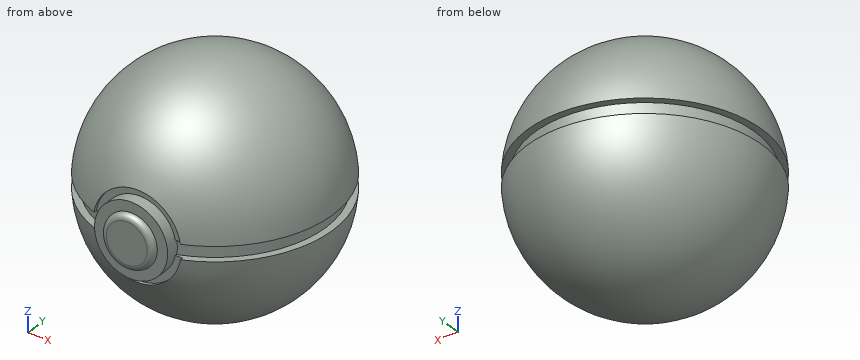
from build123d import *

# Parameters (mm, degrees)
F2_R     = 12.5
F3_DEPTH = 40
F4_R     = 15
F4_R_2   = 12.5
F5_DEPTH = 4
F6_R     = 9
F7_DEPTH = 2
F8_R     = 1.99999


# Not quite as in the source:
# - a fillet or chamfer is up to 0.001 mm smaller than in the source, because OpenCascade refuses the exact size


with BuildPart() as f1:
    # F0 (on Front) → F1 (revolve)
    with BuildSketch(Plane.XZ):
        with BuildLine():
            Line((0, 40), (0, -40))
            ThreePointArc((0, -40), (27.3861278753, -29.1547594742), (39.9217985567, -2.5))
            Line((39.9217985567, -2.5), (37.5, -2.5))
            Line((37.5, -2.5), (37.5, 0))
            Line((37.5, 0), (37.5, 2.5))
            Line((37.5, 2.5), (39.9217985567, 2.5))
            ThreePointArc((39.9217985567, 2.5), (27.3861278753, 29.1547594742), (0, 40))
        make_face()
    revolve(axis=Axis((0, 0, 0), (0, 0, -1)))

    # F2 (on Front) → F3 (join)
    with BuildSketch(Plane.XZ):
        Circle(F2_R)
    extrude(amount=F3_DEPTH)

    # F4 (on face) → F5 (cut)
    with BuildSketch(Plane.XZ.offset(40)):
        Circle(F4_R)
        Circle(F4_R_2, mode=Mode.SUBTRACT)
    extrude(amount=-F5_DEPTH, mode=Mode.SUBTRACT)

    # F6 (on face) → F7 (join)
    with BuildSketch(Plane.XZ.offset(40)):
        Circle(F6_R)
    extrude(amount=F7_DEPTH)

    # F8 (radius 2 in the source; OpenCascade refuses exactly that, so slightly less here)
    f8_edges = [f1.edges().sort_by_distance(p)[0] for p in [
        (-9, -42, 0),
    ]]
    fillet(f8_edges, radius=F8_R)


solid = f1.part
Geometry check sheet. Reference: the model listing, model coordinates, mm. Give positions to 0.01 mm unless a question says otherwise; leave off trailing zeros. Loops run counter-clockwise (first coordinate to the right, second up) from the corner with the lowest first, then second, coordinate; pieces in that order, holes last. Notation, with made-up numbers: M 67.25,12.5 L 92.25,12.5 A12 cw 92.25,26.5 Z; hole C -9,53 d8. An arc over 180 degrees is marked long. Write each question's results on one line, items separated by ' | '.
1) Section check D-D, the plane y = 16. Record the boundary of the cut face in (x, z).
Answers follow:
outline: M -36.58,-2.5 A36.66 ccw 36.58,-2.5 L 33.92,-2.5 L 33.92,2.5 L 36.58,2.5 A36.66 ccw -36.58,2.5 L -33.92,2.5 L -33.92,-2.5 Z
2) Section check B-B, the plane y = 0. Record the boundary of the cut face in (x, z), plus the area to 3 significant figures.
Answers follow:
outline: M -39.92,-2.5 A40 ccw 39.92,-2.5 L 37.5,-2.5 L 37.5,2.5 L 39.92,2.5 A40 ccw -39.92,2.5 L -37.5,2.5 L -37.5,-2.5 Z | area: 5,000 mm2
3) Gauge pin test, flat ends, axial feed: pin 1 (10 mm diameter, centred on x = -28.5, z = -28, fed in from +Y); pin 2 (4 mm diameter, centred on x = 5.5, y = 8.5, fed in from +Z); pin 3 (1 mm diameter, centred on x = 26.5, z = -18, fed in from -Y). Record the tip position at first contact, or that the pin passes through.
Answers follow:
pin 1: y = 19.45 | pin 2: z = 39.17 | pin 3: y = -24.61
4) Thickness scan on line 1 (X direction, y = -30, z = 14.5); line 2 (Y direction, x = 3, z = -22); line 3 (X direction, y = 6, z = 23). Record the ranges inside material, lowest first.
Answers follow:
line 1: -22.13 to 22.13 | line 2: -33.27 to 33.27 | line 3: -32.17 to 32.17
